```python
from build123d import *

# Parameters (mm, degrees)
SKETCH1_W           = 142.5
SKETCH1_H           = 56.74
BOSS_EXTRUDE1_DEPTH = 3
CUT_EXTRUDE1_DEPTH  = 77.749067747
SKETCH3_W           = 2.425
SKETCH3_H           = 56.74
CUT_EXTRUDE2_DEPTH  = 77.749067747
SKETCH4_W           = 65
SKETCH4_H           = 8
SKETCH4_H_2         = 56.74
BOSS_EXTRUDE2_DEPTH = 5.5
FILLET1_R           = 10
SKETCH5_R           = 2.15
CUT_EXTRUDE3_DEPTH  = 81.18472049
BOSS_EXTRUDE5_DEPTH = 5.5
CHAMFER6_SIZE       = 3
SKETCH11_R          = 2.15
CUT_EXTRUDE5_DEPTH  = 109.425008762


with BuildPart() as part:
    # Sketch1 → Boss-Extrude1 (new body)
    with BuildSketch(Plane.XY):
        Rectangle(SKETCH1_W, SKETCH1_H)
    extrude(amount=BOSS_EXTRUDE1_DEPTH)

    # Sketch2 → Cut-Extrude1 (cut, through all)
    with BuildSketch(Plane.XY.offset(3)):
        Polygon((67.771628048, 28.37), (71.25, 0), (71.25, 28.37), align=None)
        Polygon((71.25, -28.37), (71.25, 0), (67.771628048, -28.37), align=None)
    extrude(amount=-CUT_EXTRUDE1_DEPTH, mode=Mode.SUBTRACT)

    # Sketch3 → Cut-Extrude2 (cut, through all)
    with BuildSketch(Plane.XY.offset(3)):
        with Locations((-70.0375, 0)):
            Rectangle(SKETCH3_W, SKETCH3_H)
    extrude(amount=-CUT_EXTRUDE2_DEPTH, mode=Mode.SUBTRACT)

    # Sketch4 → Boss-Extrude2 (add)
    with BuildSketch(Plane.XY.offset(3)):
        with Locations((-36.325, 32.37)):
            Rectangle(SKETCH4_W, SKETCH4_H)
        with Locations((-36.325, 0)):
            Rectangle(SKETCH4_W, SKETCH4_H_2)
        with Locations((-36.325, -32.37)):
            Rectangle(SKETCH4_W, SKETCH4_H)
    extrude(amount=-BOSS_EXTRUDE2_DEPTH)

    # Fillet1
    # the kernel refuses this fillet: 10 mm, written as the material it adds along each edge
    with BuildSketch(Plane(origin=(-3.825, 28.37, 0), x_dir=(1, 0, 0), z_dir=(0, -1, 0))) as fillet1_piece_1:
        with BuildLine():
            CenterArc((6.614378278, -10), FILLET1_R, 90, 41.409622109)
            Line((0, -2.5), (-0.132287566, -2.35))
            ThreePointArc((-0.132287566, -2.35), (-0.2, -1.25), (-0.2, 0))
            Line((-0.2, 0), (0, 0.2))
            Line((0, 0.2), (6.614378278, 0.2))
            Line((6.614378278, 0.2), (6.614378278, 0))
        make_face()
    extrude(amount=56.74)

    # Sketch5 → Cut-Extrude3 (cut, through all)
    with BuildSketch(Plane.XY.offset(3)):
        with Locations((60.808027892, 17)):
            Circle(SKETCH5_R)
        with Locations((60.808027892, -17)):
            Circle(SKETCH5_R)
        with Locations((45.808027892, 17)):
            Circle(SKETCH5_R)
        with Locations((45.808027892, -17)):
            Circle(SKETCH5_R)
    extrude(amount=-CUT_EXTRUDE3_DEPTH, mode=Mode.SUBTRACT)

    # Sketch10 → Boss-Extrude5 (add)
    with BuildSketch(Plane.XY.offset(3)):
        Polygon((-68.825, 36.37), (-33.825, 36.37), (-33.825, 51.37), (-68.825, 51.37), (-95.325, 51.37), (-95.325, -51.37), (-68.825, -51.37), (-33.825, -51.37), (-33.825, -36.37), (-68.825, -36.37), align=None)
    extrude(amount=-BOSS_EXTRUDE5_DEPTH)

    # Chamfer6
    chamfer6_edges = [part.edges().sort_by_distance(p)[0] for p in [
        (-18.825, 36.37, 3),
        (-18.825, -36.37, 3),
        (-33.825, 43.87, 3),
        (-64.575, 51.37, 3),
        (-64.575, -51.37, 3),
        (-33.825, -43.87, 3),
        (-3.825, 32.37, 3),
        (-3.825, -32.37, 3),
    ]]
    chamfer(chamfer6_edges, length=CHAMFER6_SIZE)

    # Sketch11 → Cut-Extrude5 (cut, through all)
    with BuildSketch(Plane.XY.offset(3)):
        with Locations((-62.71489096, -43.079989287)):
            Circle(SKETCH11_R)
        with Locations((-54.714891019, -33.183924722)):
            Circle(SKETCH11_R)
        with Locations((-23.821377075, -30.196715875)):
            Circle(SKETCH11_R)
    cut_extrude5 = extrude(amount=-CUT_EXTRUDE5_DEPTH, mode=Mode.SUBTRACT)

    # Mirror2: Cut-Extrude5 across plane
    add(cut_extrude5.mirror(Plane.ZX), mode=Mode.SUBTRACT)


solid = part.part
```
For this review, take the finished solid that the model builds, in its own axes (mm). A direction names the side the tool comes from. Give positions to 0.01 mm unless a question says otherwise; leave off trailing zeros. Write each loop counter-clockwise with the first axis right and the second up, starting at its lowest first coordinate (ties: lowest second). Pieces come first, ordered by that corner, then holes.
Item 1: The part is to be moulded in two halves that separate along X. For faces 1 (the face through (-5.304, 31.425, 1.479)), 2 (the face through (-60.664, -42.434, 0.288)), 3 (the face through (-50, 1, -2.5)), say which applies: +X half, -X half, draft (parallel to the pull), parting line (faces both ways), or undercut.
Item 2: Take a section at D-D (y = 6.5). Give the boundary of the cut face in (x, z) (3 decimals).
Item 3: Take a section at C-C (x = -17). Give the boundary of the cut face in (y, z).
Item 4: Insertion check: P1, Ø3.5, axis at x = -23.82, y = 30.2, coming from the -Z side; P2, Ø1.5, axis at x = 17.5, z = 2.5, coming from the +Y side; P3, Ø8, axis at x = 18.5, y = 23, coming from the -Z side; P4, Ø0.8, axis at x = -24, z = -1.5, coming from the +Y side. Each pin has a flat end and moves straight along its axis. Give the tip position at first contact, or say it passes through.
Item 5: Machinability: for faces 4 (the face through (-20.56, 34.85, 1.52)), 5 (the face through (37, 0, 0)), 6 (the face through (69.535, -13.986, 1.521)), 7 (the face through (69.486, 14.384, 1.521)), 8 (the face through (-5.304, -31.537, 1.479)), which of the approach directions +Z, -Z, +X, -X, +Y, -Y give a long, thin tool a straight path to every point of the face, cutting with its end or side? Answer none if there is none.
Item 6: Take a section at A-A (z = 1.05). Give the number of separate pieces and of enclosed holes in the cut face, and give its area (3 significant figures).
Item 7: Take a section at B-B (y = -17). Give the boundary of the cut face in (x, z) (3 decimals).
Item 8: Wall thickness on probe 1 along Y at (x, z) = (-56, -1.6); probe 2 along Y at (x, z) = (20, 2.6); probe 3 along X at (y, z) = (29.5, -1.6) (3 decimals): over which ranges is each line inside the solid? List them lowest first.
Established:
1. face 1: +X half
1. face 2: undercut
1. face 3: draft
2. outline: (-95.325, -2.5) - (-3.825, -2.5) arc R10 cw to (2.789, 0) - (70.453, 0) - (70.453, 3) - (-95.325, 3) - close
3. outline: (-36.37, -2.5) - (36.37, -2.5) - (36.37, 0) - (33.37, 3) - (-33.37, 3) - (-36.37, 0) - close
4. P1: passes through
4. P2: stops at y = 28.37
4. P3: stops at z = 0
4. P4: stops at y = 36.37
5. face 4: +Z, +X, +Y
5. face 5: -Z, +X, +Y, -Y
5. face 6: +Z, -Z, +X, -Y
5. face 7: +Z, -Z, +X, +Y
5. face 8: +Z, +X, -Y
6. separate pieces: 1
6. enclosed holes: 10
6. area: 12,300 mm2
7. outline: (-95.325, -2.5) - (-3.825, -2.5) arc R10 cw to (2.789, 0) - (43.658, 0) - (43.658, 3) - (-95.325, 3) - close; (47.958, 0) - (58.658, 0) - (58.658, 3) - (47.958, 3) - close; (62.958, 0) - (69.166, 0) - (69.166, 3) - (62.958, 3) - close
8. probe 1: y = -51.37 to -34.91, -31.46 to 31.46, 34.91 to 51.37
8. probe 2: y = -28.37 to 28.37
8. probe 3: x = -95.325 to -25.855, -21.787 to -3.825
